For this review, take the finished solid that the model builds, in its own axes (mm). A direction names the side the tool comes from. Round coordinates to 2 decimals unless told otherwise and drop trailing zeros. Loops run counter-clockwise (first coordinate to the right, second up) from the corner with the lowest first, then second, coordinate; pieces in that order, holes last.
```python
from build123d import *

# Parameters (mm, degrees)
BOSS_EXTRUDE1_DEPTH = 3.175
FILLET1_R           = 12.7
SKETCH2_R           = 0.85
SKETCH2_W           = 12
SKETCH2_H           = 1.7
CUT_EXTRUDE1_DEPTH  = 41.783613437
SKETCH3_W           = 2.286
SKETCH3_H           = 20.32
SKETCH3_W_2         = 12.7
SKETCH3_H_2         = 11.43
SKETCH3_W_3         = 6.35
SKETCH3_H_3         = 2.54
CUT_EXTRUDE2_DEPTH  = 41.783613437


with BuildPart() as part:
    # Sketch1 → Boss-Extrude1 (new body)
    with BuildSketch(Plane.XY):
        Polygon((19.05, -25.4), (-19.05, -25.4), (-19.05, -19.685), (-31.75, -19.685), (-31.75, -13.335), (-19.05, -13.335), (-19.05, 25.4), (19.05, 25.4), (19.05, -13.335), (31.75, -13.335), (31.75, -19.685), (19.05, -19.685), align=None)
    extrude(amount=BOSS_EXTRUDE1_DEPTH)

    # Fillet1
    fillet1_edges = [part.edges().sort_by_distance(p)[0] for p in [
        (-19.05, 25.4, 1.5875),
        (19.05, 25.4, 1.5875),
    ]]
    fillet(fillet1_edges, radius=FILLET1_R)

    # Sketch2 → Cut-Extrude1 (cut, through all)
    with BuildSketch(Plane.XY):
        with Locations((0, 5.364988)):
            Circle(SKETCH2_R)
        with Locations((-3.302, 5.364988)):
            Circle(SKETCH2_R)
        with Locations(Location((3.302, 5.364988, 0), (0, 0, 180))):
            Circle(SKETCH2_R)
        with Locations((0, 0.864988)):
            Rectangle(SKETCH2_W, SKETCH2_H)
        with Locations((0, 9.864988)):
            Rectangle(SKETCH2_W, SKETCH2_H)
    extrude(amount=CUT_EXTRUDE1_DEPTH, mode=Mode.SUBTRACT)

    # Sketch3 → Cut-Extrude2 (cut, through all)
    with BuildSketch(Plane.XY):
        with Locations((-12.4167697, -15.24)):
            Rectangle(SKETCH3_W, SKETCH3_H)
        with Locations((0, -8.240012)):
            Rectangle(SKETCH3_W_2, SKETCH3_H_2)
        with Locations((-12.4167697, -12.7)):
            Rectangle(SKETCH3_W_3, SKETCH3_H_3)
        with Locations((12.4167697, -12.7)):
            Rectangle(SKETCH3_W_3, SKETCH3_H_3)
        with Locations((12.4167697, -15.24)):
            Rectangle(SKETCH3_W, SKETCH3_H)
    extrude(amount=CUT_EXTRUDE2_DEPTH, mode=Mode.SUBTRACT)


solid = part.part
```
(1) For faces 1 (the flat face through (11.274, -20, 2)), 2 (the flat face through (0, -13.955, 2)), 3 (the flat face through (16, -25.4, 2)), 4 (the flat face through (-25, -19.685, 2)), 5 (the flat face through (19.05, 0, 2)), list the 3-axis set-ups (+Z, -Z, +X, -X, +Y, -Y) from which the entire face can be reached by the end or side of a thin tool; tool diameter is ignored.
(2) Add section B-B (y = -21). Give the boundary of the cut face in (x, z) (3 decimals), plus the area to 3 significant figures.
(3) Add section A-A (x = 0). Give the boundary of the cut face in (y, z) (3 decimals).
(4) Add section C-C (y = -7.5). Give the boundary of the cut face in (x, z) (3 decimals), plus the area to 3 significant figures.
(5) The part is to be moulded in two halves that separate along X. For faces 6 (the flat face through (0, 9.015, 2)), 7 (the flat face through (31.75, -16, 2)), 8 (the flat face through (-19.05, 0, 2)), 9 (the flat face through (-7, 0, 3.175)), say which applies: pulls with the +X half, pulls with the -X half, needs draft (parallel to the pull), parting line crosses it, or undercut.
(6) For L1, parallel to X at y = -23, z = 0.9; L2, parallel to Y at x = 0, z = 1.05; L3, parallel to Y at x = 2, z = 0.9, list the stretches that pass through material, from the lowest coordinate up.
(7) Insertion check: pin 1 Ø1.8 at (x, z) = (-12, 2) entering from -Y; pin 2 Ø1 at (x, z) = (23, 2.5) entering from +Y (3 decimals); pin 3 Ø1 at (x, z) = (25, 2) entering from -Y (3 decimals); pin 4 Ø1.5 at (x, z) = (16, 0.5) entering from +Y. Each pin has a flat end and moves straight along its axis. Give the tip position at first contact, or say it passes through.
(8) Add section D-D (x = 22). Give the boundary of the cut face in (y, z) (3 decimals).
Outcome:
1. face 1: +Z, -Z, -Y
1. face 2: +Z, -Z
1. face 3: +Z, -Z, +X, -X, -Y
1. face 4: +Z, -Z, -X, -Y
1. face 5: +Z, -Z, +X, +Y
2. outline: (-19.05, 0) - (-13.56, 0) - (-13.56, 3.175) - (-19.05, 3.175) - close; (-11.274, 0) - (11.274, 0) - (11.274, 3.175) - (-11.274, 3.175) - close; (13.56, 0) - (19.05, 0) - (19.05, 3.175) - (13.56, 3.175) - close
2. area: 106 mm2
3. outline: (-25.4, 0) - (-13.955, 0) - (-13.955, 3.175) - (-25.4, 3.175) - close; (-2.525, 0) - (0.015, 0) - (0.015, 3.175) - (-2.525, 3.175) - close; (1.715, 0) - (4.515, 0) - (4.515, 3.175) - (1.715, 3.175) - close; (6.215, 0) - (9.015, 0) - (9.015, 3.175) - (6.215, 3.175) - close; (10.715, 0) - (25.4, 0) - (25.4, 3.175) - (10.715, 3.175) - close
4. outline: (-19.05, 0) - (-13.56, 0) - (-13.56, 3.175) - (-19.05, 3.175) - close; (-11.274, 0) - (-6.35, 0) - (-6.35, 3.175) - (-11.274, 3.175) - close; (6.35, 0) - (11.274, 0) - (11.274, 3.175) - (6.35, 3.175) - close; (13.56, 0) - (19.05, 0) - (19.05, 3.175) - (13.56, 3.175) - close
4. area: 66.1 mm2
5. face 6: undercut
5. face 7: pulls with the +X half
5. face 8: pulls with the -X half
5. face 9: needs draft
6. L1: x = -19.05 to -13.56, -11.27 to 11.27, 13.56 to 19.05
6. L2: y = -25.4 to -13.96, -2.53 to 0.01, 1.71 to 4.51, 6.21 to 9.01, 10.71 to 25.4
6. L3: y = -25.4 to -13.96, -2.53 to 0.01, 1.71 to 9.01, 10.71 to 25.4
7. pin 1: stops at y = -25.4
7. pin 2: stops at y = -13.335
7. pin 3: stops at y = -19.685
7. pin 4: stops at y = 21.76
8. outline: (-19.685, 0) - (-13.335, 0) - (-13.335, 3.175) - (-19.685, 3.175) - close
